Can you work these out from the drawing? Everything is in mm from the part's minimum corner. Give positions to 0.01 mm unless a question says otherwise; leave off trailing zeros. Order: outer loops, then holes, each group sorted by start corner. A loop starts at its lowest first (then second) coordinate and runs counter-clockwise, first axis right, second up. Notation, with made-up numbers: M 64.5,-26.5 L 119.5,-26.5 A15 ccw 119.5,-6.5 Z; hole C -24,-15.5 d5. An arc over 180 degrees is marked long. Use a Markdown table: item, result. Add a question column.
Item 1: Suppose I cut it at B-B on z = 18.5. Write out the boundary of the cut face in (x, y).
Item 2: I'm going to push flat-ended pins straight in: pin 1 Ø1.6 at (x, y) = (12.5, 1.5) entering from -Z; pin 2 Ø1.6 at (y, z) = (2, 3) entering from +X; pin 3 Ø3 at (y, z) = (3, 4) entering from -X; pin 4 Ø8 at (x, z) = (110, 26.5) entering from -Y. Where does each tip first touch, or does it pass through?
Item 3: Suppose I cut it at A-A on x = 190. Write out the boundary of the cut face in (y, z).
Item 4: Suppose I cut it at D-D on x = 26. Write out the boundary of the cut face in (y, z).
Item 5: Suppose I cut it at C-C on y = 3.65. Write out the boundary of the cut face in (x, z), plus the area to 3 significant figures.
Item 6: If I drill on L1, parallel to X at y = 2.5, z = 18.5; L2, parallel to Z at x = 190, y = 4.25; L3, parallel to X at y = 5.25, z = 4, over which ranges is the centre line in solid material (lowest first)? Write a range as from..to.
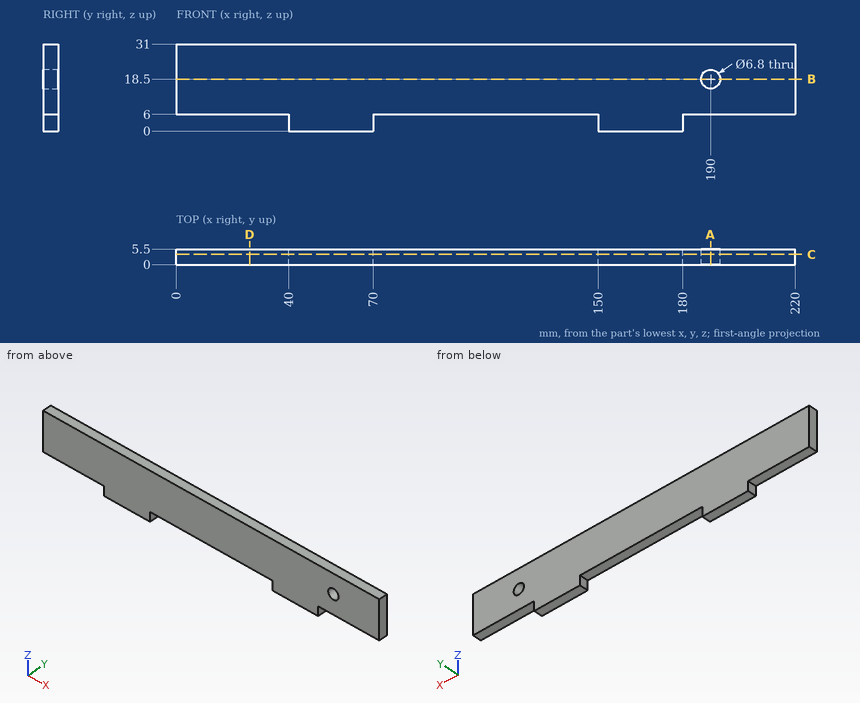
Findings below:
| question | item | result |
|---|---|---|
| 1 | outline | M 0,0 L 186.6,0 L 186.6,5.5 L 0,5.5 Z; M 193.4,0 L 220,0 L 220,5.5 L 193.4,5.5 Z |
| 2 | pin 1 | stops at z = 6 |
| 2 | pin 2 | stops at x = 180 |
| 2 | pin 3 | stops at x = 40 |
| 2 | pin 4 | stops at y = 0 |
| 3 | outline | M 0,6 L 5.5,6 L 5.5,15.1 L 0,15.1 Z; M 0,21.9 L 5.5,21.9 L 5.5,31 L 0,31 Z |
| 4 | outline | M 0,6 L 5.5,6 L 5.5,31 L 0,31 Z |
| 5 | outline | M 0,6 L 40,6 L 40,0 L 70,0 L 70,6 L 150,6 L 150,0 L 180,0 L 180,6 L 220,6 L 220,31 L 0,31 Z; hole C 190,18.5 d6.8 |
| 5 | area | 5,820 mm^2 |
| 6 | L1 | x = 0..186.6, 193.4..220 |
| 6 | L2 | z = 6..15.1, 21.9..31 |
| 6 | L3 | x = 40..70, 150..180 |
